CAD build for the part. Positions are in the model's coordinates, mm. A direction names the side the tool comes from. Round coordinates to 2 decimals unless told otherwise and drop trailing zeros. Loops run counter-clockwise (first coordinate to the right, second up) from the corner with the lowest first, then second, coordinate; pieces in that order, holes last. Notation, with made-up numbers: (40, 16.25) -> (83, 16.25) arc R19 ccw to (83, 51.25) -> close; hole circle Ø7 at (16, -22). An arc over 180 degrees is marked (long way). Answer as CSV lines item,"result".
Autodesk Inventor part; units mm, degrees
ref_plane "YZ Plane" through (0, 0, 0) normal (1, 0, 0) x (0, 1, 0)
ref_plane "XZ Plane" through (0, 0, 0) normal (0, 1, 0) x (-1, 0, 0)
ref_plane "XY Plane" through (0, 0, 0) normal (0, 0, 1) x (1, 0, 0)
sketch "Sketch1" plane through (0, 0, 0) normal (0, 0, 1) x (1, 0, 0)
  line L0 (-50, 50) -> (50, 50)
  line L1 (50, 50) -> (50, -50)
  line L2 (50, -50) -> (-50, -50)
  line L3 (-50, -50) -> (-50, 50)
  line L4 (-50, 50) -> (50, -50) construction
  line L5 (50, 50) -> (-50, -50) construction
  line L6 (0, 50) -> (0, -50) construction
  circle A0 centre (-35, -35) radius 6.5
  circle A1 centre (-35, 35) radius 6.5
  circle A2 centre (35, -35) radius 6.5
  circle A3 centre (35, 35) radius 6.5
  line L7 (35, 35) -> (-35, 35) construction
  line L8 (-35, 35) -> (-35, -35) construction
  line L9 (-35, -35) -> (35, -35) construction
  line L10 (35, -35) -> (35, 35) construction
  line L11 (35, 35) -> (-35, -35) construction
  line L12 (-35, 35) -> (35, -35) construction
  point P0 (0, 0)
  dimension "d0" = 100
  dimension "d1" = 100
  dimension "d19" = 13
  dimension "d20" = 70
extrude "Plate1" add sketch "Sketch1" along normal blind 4
sketch "Sketch3" plane through (50, -54, 0) normal (0, 1, 0) x (-1, 0, 0)
  line L0 (100, 0) -> (0, 0)
  line L1 (0, 0) -> (0, 25)
  line L2 (0, 25) -> (100, 25)
  line L3 (100, 25) -> (100, 0)
edge flange "Flange1" height 25 angle 90 thickness 4 bend radius 4 thickness toward (0, 1, 0) relief tear relief width 4 relief depth 2 corner gap 4 corner form 0 edges at (0, -50, 4) (0, 50, 4) wall of the first edge with corners at (-50, -54, 0) (50, -54, 0) (50, -54, 25) (-50, -54, 25)
bend "Bend1"
corner "Corner1"
equation "\"d0\" = d1"
equation "\"d2\" = Thickness"
equation "\"d21\" = BendReliefWidth"
equation "\"d22\" = BendReliefDepth"
equation "\"d23\" = MinimumRemnant"
equation "\"d24\" = TransitionRadius"
equation "\"d27\" = BendRadius"
equation "\"d28\" = CornerReliefSize"
equation "\"d29\" = GapSize"
equation "\"d30\" = JacobiRadiusSize"
equation "\"BendRadius\" = Thickness"
equation "\"BendReliefWidth\" = Thickness"
equation "\"BendReliefDepth\" = 0.5 * Thickness"
equation "\"CornerReliefSize\" = 4 * Thickness"
equation "\"MinimumRemnant\" = 2 * Thickness"
equation "\"TransitionRadius\" = BendRadius"
equation "\"JacobiRadiusSize\" = BendRadius"
equation "\"GapSize\" = Thickness"
properties part number "GBK-RK-0820 ring plate_CPY"
Q1. Probe L1, parallel to Y at x = 13.5, z = 15; L2, parallel to Y at x = -31.5, z = 1.5; L3, parallel to Y at x = 35, z = 1. List the from-to ranges inside material, lowest first. Write a range as [from, to].
Results:
L1,"[-54, -50], [50, 54]"
L2,"[-50.66, -40.48], [-29.52, 29.52], [40.48, 50.66]"
L3,"[-49.87, -41.5], [-28.5, 28.5], [41.5, 49.87]"
Q2. Two-plate mould, pull along Y, no slides. Class faces 3 (the flat face through (1, -52, 25)), 4 (the cylindrical face through (-0.7, 51.719, 2.406)), 5 (the cylindrical face through (30.209, -39.393, 1.972)): pulls with the +Y half, pulls with the -Y half, needs draft (parallel to the pull), parting line crosses it, or undercut.
Results:
face 3,"needs draft"
face 4,"pulls with the +Y half"
face 5,"undercut"
Q3. Slice it at B-B, the plane x = 37.5. Give the cut face in (y, z).
Results:
outline,"(-54, 8) arc R8 ccw to (-46, 0) -> (-41, 0) -> (-41, 4) -> (-46, 4) arc R4 cw to (-50, 8) -> (-50, 25) -> (-54, 25) -> close; (-29, 0) -> (29, 0) -> (29, 4) -> (-29, 4) -> close; (41, 0) -> (46, 0) arc R8 ccw to (54, 8) -> (54, 25) -> (50, 25) -> (50, 8) arc R4 cw to (46, 4) -> (41, 4) -> close"
Q4. Tool access for faces 1 (the flat face through (-1, 1, 4)), 2 (the flat face through (-1, 52, 25)): list every direction of +Z, -Z, +X, -X, +Y, -Y with a clear straight run to the whole face (end or side of a thin tool).
Results:
face 1,"+Z, +X, -X"
face 2,"+Z, +X, -X, +Y, -Y"
Q5. Drop a flat-ended pin along its axis: pin 1 Ø3 at (x, y) = (-29, 18.5) entering from +Z. Give the stop position or say it passes through.
Results:
pin 1,"z = 4"
Q6. Slice it at C-C, the plane y = 35. Give the cut face in (x, z), and give its area (3 significant figures).
Results:
outline,"(-50, 0) -> (-41.5, 0) -> (-41.5, 4) -> (-50, 4) -> close; (-28.5, 0) -> (28.5, 0) -> (28.5, 4) -> (-28.5, 4) -> close; (41.5, 0) -> (50, 0) -> (50, 4) -> (41.5, 4) -> close"
area,"296 mm2"
Q7. Slice it at A-A, the plane z = 23. Give the cut face in (x, y), and give its area (3 significant figures).
Results:
outline,"(-50, -54) -> (50, -54) -> (50, -50) -> (-50, -50) -> close; (-50, 50) -> (50, 50) -> (50, 54) -> (-50, 54) -> close"
area,"800 mm2"
Q8. Slice it at D-D, the plane x = 25.5. Give the cut face in (y, z).
Results:
outline,"(-54, 8) arc R8 ccw to (-46, 0) -> (46, 0) arc R8 ccw to (54, 8) -> (54, 25) -> (50, 25) -> (50, 8) arc R4 cw to (46, 4) -> (-46, 4) arc R4 cw to (-50, 8) -> (-50, 25) -> (-54, 25) -> close"
